Source: CAD feature listing. Evaluate the final solid. Frame: model axes, mm. Face numbers are marked on the shaded views. A direction names the side the tool comes from. Round coordinates to 2 decimals unless told otherwise and drop trailing zeros. Order: outer loops, then holes, each group sorted by start corner. A loop starts at its lowest first (then second) coordinate and runs counter-clockwise, first axis right, second up. Notation, with made-up numbers: (6.5, 3) -> (42.5, 3) arc R33 ccw to (42.5, 36) -> close; hole circle Ø4 at (65.5, 81). An arc over 180 degrees is marked (long way). One line per item, written item: value. Start each with the question number.
1) Mould query, pull axis X, two halves, no side actions, for the marked faces 1, 2 and 3. Classes: pulls with the +X half, pulls with the -X half, needs draft (parallel to the pull), parting line crosses it, or undercut.
2) Reachability of the marked faces 4, 5 and 6 from +Z, -Z, +X, -X, +Y, -Y: full face, straight path, thin tool, end or side. Return the list, or none.
3) Section A-A (z = 68). State how many separate pieces and enclosed holes the cut face has, and give its area (3 significant figures).
4) Ray query, L1, parallel to Y at x = -35.5, z = 53 (1 decimal); L2, parallel to Z at x = 23, y = 23.5; L3, parallel to Y at x = -33, z = 18 (1 decimal). Return the intervals inside material, ascending.
5) Section B-B (x = -21). Return the cut outline in (y, z) (1 decimal).
6) Pin query (flat end, axial travel): P1, Ø5, axis at x = -49.5, y = -35.5, coming from the +Z side; P2, Ø8, axis at x = -0.5, y = -12.5, coming from the -Z side; P3, Ø16.5, axis at x = 6, y = 36, coming from the +Z side; P4, Ø2.5, axis at x = -37.5, z = 7.5, coming from the -Y side. Return the tip coordinate at first contact, or that it passes through.
```python
from build123d import *

# Parameters (mm, degrees)
F0_W      = 114.3
F0_H      = 101.6
F1_DEPTH  = 1.5875
F2_W      = 46.355
F2_H      = 46.355
F2_W_2    = 43.18
F2_H_2    = 43.18
F3_DEPTH  = 45.72
F4_W      = 88.9
F4_H      = 1.5875
F5_DEPTH  = 45.72
F7_DEPTH  = 88.9
F9_DEPTH  = 1.5875
F11_DEPTH = 1.5875
F12_W     = 25.4
F12_H     = 27.6225
F12_W_2   = 22.225
F12_H_2   = 24.4475
F12_W_3   = 7.874
F12_H_3   = 15.367
F12_W_4   = 4.699
F12_H_4   = 12.192
F13_DEPTH = 15.875
F14_W     = 25.4
F14_H     = 27.6225
F14_W_2   = 4.699
F14_H_2   = 12.192
F15_DEPTH = 1.5875
F17_DEPTH = 25.4
F18_W     = 6.35
F18_H     = 21.59
F19_DEPTH = 38.1
F21_DEPTH = 27.94
F23_DEPTH = 25.4
F25_DEPTH = 3.175
F26_R     = 31.75
F27_DEPTH = 3.175
F28_R     = 13.0175
F29_DEPTH = 27.94
F30_W     = 46.355
F30_H     = 27.6225
F30_W_2   = 43.18
F30_H_2   = 24.4475
F31_DEPTH = 76.2
F32_W     = 46.355
F32_H     = 12.7
F33_DEPTH = 1.5875
F34_W     = 43.18
F34_H     = 1.5875
F35_DEPTH = 76.2
F36_W     = 46.355
F36_H     = 12.7
F36_W_2   = 43.18
F36_H_2   = 9.525
F37_DEPTH = 38.1
F38_W     = 43.18
F38_H     = 9.525
F39_DEPTH = 25.4
F41_DEPTH = 67.945
F43_DEPTH = 25.4


with BuildPart() as f1:
    # F0 (on Top) → F1 (new body)
    with BuildSketch(Plane.XY):
        Rectangle(F0_W, F0_H)
    extrude(amount=F1_DEPTH)

    # F2 (on face) → F3 (join)
    with BuildSketch(Plane.XY.offset(1.5875)):
        with Locations((-33.9725, 0)):
            Rectangle(F2_W, F2_H)
        with Locations((-33.9725, 0)):
            Rectangle(F2_W_2, F2_H_2, mode=Mode.SUBTRACT)
    extrude(amount=F3_DEPTH)

    # F4 (on face) → F5 (join)
    with BuildSketch(Plane.XY.offset(1.5875)):
        with Locations((12.7, -22.38375)):
            Rectangle(F4_W, F4_H)
    extrude(amount=F5_DEPTH)

    # F6 (on face) → F7 (join)
    with BuildSketch(Plane.YZ.offset(57.15)):
        Polygon((-23.1775, 47.3075), (-39.818219, 1.5875), (-38.128837, 1.5875), (-23.1775, 42.665961), align=None)
        Polygon((-46.456344, 13.521596), (-50.8, 1.5875), (-39.818219, 1.5875), (-48.023614, 4.574019), (-44.964582, 12.978639), align=None)
    extrude(amount=-F7_DEPTH)

    # F8 (on face) → F9 (join)
    with BuildSketch(Plane.YZ.offset(57.15)):
        Polygon((-23.1775, 1.5875), (-23.1775, 42.665961), (-38.128837, 1.5875), align=None)
    extrude(amount=-F9_DEPTH)

    # F10 (on face) → F11 (join)
    with BuildSketch(Plane(origin=(-31.75, 0, 0), x_dir=(0, -1, 0), z_dir=(-1, 0, 0))):
        Polygon((23.1775, 1.5875), (38.128837, 1.5875), (23.1775, 42.665961), align=None)
    extrude(amount=-F11_DEPTH)

    # F12 (on face) → F13 (join)
    with BuildSketch(Plane.XY.offset(1.5875)):
        with Locations((-44.45, -36.98875)):
            Rectangle(F12_W, F12_H)
        with Locations((-44.45, -36.98875)):
            Rectangle(F12_W_2, F12_H_2, mode=Mode.SUBTRACT)
        with Locations((-38.1, -34.6075)):
            Rectangle(F12_W_3, F12_H_3)
        with Locations((-38.1, -34.6075)):
            Rectangle(F12_W_4, F12_H_4, mode=Mode.SUBTRACT)
        with Locations((-50.8, -34.6075)):
            Rectangle(F12_W_3, F12_H_3)
        with Locations((-50.8, -34.6075)):
            Rectangle(F12_W_4, F12_H_4, mode=Mode.SUBTRACT)
    extrude(amount=F13_DEPTH)

    # F14 (on face) → F15 (join)
    with BuildSketch(Plane.XY.offset(17.4625)):
        with Locations((-44.45, -36.98875)):
            Rectangle(F14_W, F14_H)
        with Locations((-50.8, -34.6075)):
            Rectangle(F14_W_2, F14_H_2, mode=Mode.SUBTRACT)
        with Locations((-38.1, -34.6075)):
            Rectangle(F14_W_2, F14_H_2, mode=Mode.SUBTRACT)
    extrude(amount=-F15_DEPTH)

    # F16 (on face) → F17 (cut)
    with BuildSketch(Plane.YZ.offset(-31.75)):
        Polygon((-50.8, 17.4625), (-50.8, 1.5875), (-45.021973, 17.4625), align=None)
    extrude(amount=-F17_DEPTH, mode=Mode.SUBTRACT)

    # F18 (on face) → F19 (join)
    with BuildSketch(Plane.XY.offset(1.5875)):
        Polygon((-10.795, -18.415), (-10.795, -21.59), (57.15, -21.59), (57.15, -18.415), (50.8, -18.415), align=None)
        with Locations((53.975, -7.62)):
            Rectangle(F18_W, F18_H)
        Polygon((50.8, 3.175), (57.15, 3.175), (57.15, 6.35), (-10.795, 6.35), (-10.795, 3.175), align=None)
    extrude(amount=F19_DEPTH)

    # F20 (on face) → F21 (join, through all)
    with BuildSketch(Plane(origin=(0, -21.59, 0), x_dir=(-1, 0, 0), z_dir=(0, 1, 0))):
        Polygon((-55.353949, 41.701449), (-57.15, 43.4975), (-57.15, 39.6875), (-50.8, 39.6875), (-50.8, 41.701449), align=None)
    extrude(amount=F21_DEPTH)

    # F22 (on face) → F23 (cut)
    with BuildSketch(Plane.YZ.offset(57.15)):
        Polygon((-20.32, 43.4975), (-21.59, 43.4975), (-20.955, 42.397648), align=None)
        Polygon((6.35, 43.4975), (5.08, 43.4975), (5.715, 42.397648), align=None)
        Polygon((5.08, 43.4975), (3.81, 43.4975), (4.445, 42.397648), align=None)
        Polygon((3.81, 43.4975), (2.54, 43.4975), (3.175, 42.397648), align=None)
        Polygon((2.54, 43.4975), (1.27, 43.4975), (1.905, 42.397648), align=None)
        Polygon((1.27, 43.4975), (0, 43.4975), (0.635, 42.397648), align=None)
        Polygon((0, 43.4975), (-1.27, 43.4975), (-0.635, 42.397648), align=None)
        Polygon((-1.27, 43.4975), (-2.54, 43.4975), (-1.905, 42.397648), align=None)
        Polygon((-2.54, 43.4975), (-3.81, 43.4975), (-3.175, 42.397648), align=None)
        Polygon((-3.81, 43.4975), (-5.08, 43.4975), (-4.445, 42.397648), align=None)
        Polygon((-5.08, 43.4975), (-6.35, 43.4975), (-5.715, 42.397648), align=None)
        Polygon((-6.35, 43.4975), (-7.62, 43.4975), (-6.985, 42.397648), align=None)
        Polygon((-7.62, 43.4975), (-8.89, 43.4975), (-8.255, 42.397648), align=None)
        Polygon((-8.89, 43.4975), (-10.16, 43.4975), (-9.525, 42.397648), align=None)
        Polygon((-10.16, 43.4975), (-11.43, 43.4975), (-10.795, 42.397648), align=None)
        Polygon((-11.43, 43.4975), (-12.7, 43.4975), (-12.065, 42.397648), align=None)
        Polygon((-12.7, 43.4975), (-13.97, 43.4975), (-13.335, 42.397648), align=None)
        Polygon((-13.97, 43.4975), (-15.24, 43.4975), (-14.605, 42.397648), align=None)
        Polygon((-15.24, 43.4975), (-16.51, 43.4975), (-15.875, 42.397648), align=None)
        Polygon((-16.51, 43.4975), (-17.78, 43.4975), (-17.145, 42.397648), align=None)
        Polygon((-17.78, 43.4975), (-19.05, 43.4975), (-18.415, 42.397648), align=None)
        Polygon((-19.05, 43.4975), (-20.32, 43.4975), (-19.685, 42.397648), align=None)
    extrude(amount=-F23_DEPTH, mode=Mode.SUBTRACT)

    # F24 (on face) → F25 (join)
    with BuildSketch(Plane(origin=(0, 6.35, 0), x_dir=(-1, 0, 0), z_dir=(0, 1, 0))):
        with BuildLine():
            Line((-52.06352, 39.6875), (10.15352, 39.6875))
            ThreePointArc((10.15352, 39.6875), (-20.955, 65.0875), (-52.06352, 39.6875))
        make_face()
    extrude(amount=-F25_DEPTH)

    # F26 (on face) → F27 (join)
    with BuildSketch(Plane(origin=(0, -21.59, 0), x_dir=(-1, 0, 0), z_dir=(0, 1, 0))):
        with Locations((-20.955, 33.3375)):
            Circle(F26_R)
    extrude(amount=F27_DEPTH)

    # F28 (on face) → F29 (cut)
    with BuildSketch(Plane(origin=(0, 6.35, 0), x_dir=(-1, 0, 0), z_dir=(0, 1, 0))):
        with Locations((-20.955, 33.3375)):
            Circle(F28_R)
    extrude(amount=-F29_DEPTH, mode=Mode.SUBTRACT)

    # F30 (on face) → F31 (join)
    with BuildSketch(Plane.XY.offset(1.5875)):
        with Locations((-33.9725, 36.98875)):
            Rectangle(F30_W, F30_H)
        with Locations((-33.9725, 36.98875)):
            Rectangle(F30_W_2, F30_H_2, mode=Mode.SUBTRACT)
    extrude(amount=F31_DEPTH)

    # F32 (on face) → F33 (join)
    with BuildSketch(Plane.XY.offset(77.7875)):
        with Locations((-33.9725, 44.45)):
            Rectangle(F32_W, F32_H)
    extrude(amount=-F33_DEPTH)

    # F34 (on face) → F35 (join)
    with BuildSketch(Plane.XY.offset(77.7875)):
        with Locations((-33.9725, 38.89375)):
            Rectangle(F34_W, F34_H)
    extrude(amount=-F35_DEPTH)

    # F36 (on face) → F37 (join)
    with BuildSketch(Plane.XY.offset(77.7875)):
        with Locations((-33.9725, 44.45)):
            Rectangle(F36_W, F36_H)
        with Locations((-33.9725, 44.45)):
            Rectangle(F36_W_2, F36_H_2, mode=Mode.SUBTRACT)
    extrude(amount=F37_DEPTH)

    # F38 (on face) → F39 (cut)
    with BuildSketch(Plane.XY.offset(77.7875)):
        with Locations((-33.9725, 44.45)):
            Rectangle(F38_W, F38_H)
    extrude(amount=-F39_DEPTH, mode=Mode.SUBTRACT)

    # F40 (on face) → F41 (join, through all)
    with BuildSketch(Plane.YZ.offset(-10.795)):
        Polygon((26.67, 5.3975), (26.67, 1.5875), (30.48, 1.5875), (30.48, 5.3975), (34.925, 5.3975), (34.925, 7.9375), (22.225, 7.9375), (22.225, 5.3975), align=None)
    extrude(amount=F41_DEPTH)

    # F42 (on face) → F43 (join)
    with BuildSketch(Plane.YZ.offset(-31.75)):
        Polygon((-43.434473, 17.4625), (-45.021973, 17.4625), (-50.8, 1.5875), (-50.8, 0), (-49.790303, 0), align=None)
    extrude(amount=-F43_DEPTH)


solid = f1.part
```
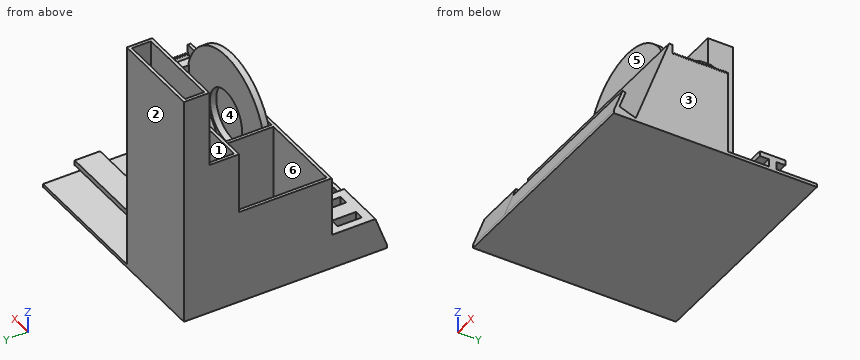
Findings:
1. face 1: undercut
1. face 2: needs draft
1. face 3: pulls with the +X half
2. face 4: +Y
2. face 5: +Z, +X, -X, -Y
2. face 6: +Z
3. separate pieces: 1
3. enclosed holes: 2
3. area: 293 mm2
4. L1: 23.2 to 24.8, 38.1 to 39.7, 49.2 to 50.8
4. L2: 0 to 1.59, 5.4 to 7.94
4. L3: -23.2 to -21.6, 21.6 to 24.8, 38.1 to 39.7, 49.2 to 50.8
5. outline: (-50.8, 0) -> (50.8, 0) -> (50.8, 115.9) -> (49.2, 115.9) -> (49.2, 1.6) -> (39.7, 1.6) -> (39.7, 115.9) -> (38.1, 115.9) -> (38.1, 1.6) -> (24.8, 1.6) -> (24.8, 77.8) -> (23.2, 77.8) -> (23.2, 47.3) -> (21.6, 47.3) -> (21.6, 1.6) -> (-21.6, 1.6) -> (-21.6, 47.3) -> (-23.2, 47.3) -> (-39.8, 1.6) -> (-48, 4.6) -> (-45, 13) -> (-46.5, 13.5) -> (-50.8, 1.6) -> close; hole (-38.1, 1.6) -> (-23.2, 1.6) -> (-23.2, 42.7) -> close
6. P1: z = 17.46
6. P2: z = 0
6. P3: z = 7.94
6. P4: y = -49.1
